Study the drawing (mm; zero at the part's minimum x, y, z) and answer. A direction names the side the tool comes from. Give positions to 0.01 mm unless a question says otherwise; leave off trailing zeros. Loops run counter-clockwise (first coordinate to the right, second up) from the corner with the lowest first, then second, coordinate; pieces in that order, holes last. Notation, with made-up numbers: (-21, -18) - (28, -18) arc R16 cw to (28, 10) - close; hole circle Ø2 at (-9.75, 46.25). An arc over 180 degrees is marked (long way). Answer in a Markdown table with one row per item. Add a question column.
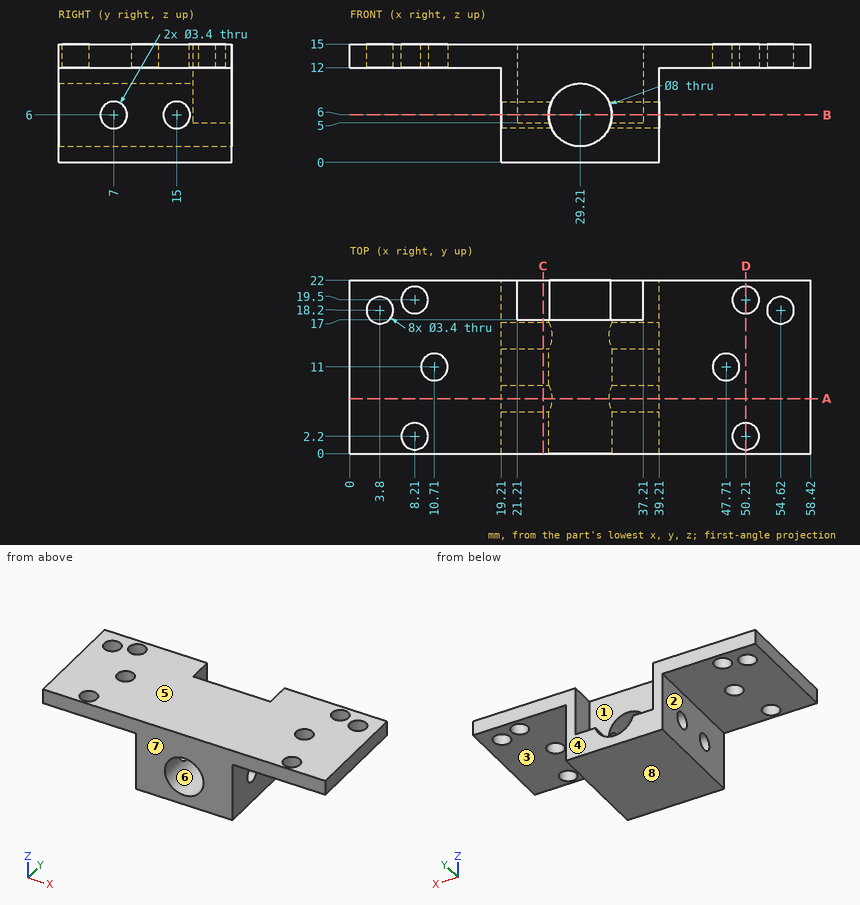
(1) A tool of negligible diameter and unlimited length cuts with its end or side. For the marked faces 1, 2, 3 and 4, from which of +Z, -Z, +X, -X, +Y, -Y can it reach the whole face along a straight path? Write none if from no direction.
(2) The mould has two halves that part along Z. Classify the marked faces 5, 6, 7 and 8: pulls with the +Z half, pulls with the -Z half, needs draft (parallel to the pull), parting line crosses it, or undercut.
(3) A cutting plane is placed at C-C on x = 24.5. Determine the outline of the cut face in (y, z), plus the area to 3 significant figures.
(4) A cutting plane is placed at B-B on z = 6. Determine the outline of the cut face in (x, y), plus the area to 3 significant figures.
(5) A cutting plane is placed at A-A on y = 7. Determine the outline of the cut face in (x, z).
(6) Find the intervals of material crossed by line 1 along Y through (x, z) = (21.5, 6); line 2 along Y through (x, z) = (8.21, 13.35); line 3 along Y through (x, z) = (3.8, 13.5), in increasing order. Write a range as [from, to].
(7) A cutting plane is placed at D-D on x = 50.21. Determine the outline of the cut face in (y, z).
(8) Given pin 1 Ø8 at (x, z) = (28.5, 9.5) entering from +Y; pin 2 Ø4 at (x, y) = (47.71, 11) entering from -Z; pin 3 Ø4 at (y, z) = (2.5, 3) entering from +X, each flat-ended and moving along its own axis, determine where each tip first touches the part or whether it passes through.
Evaluation:
| question | item | result |
|---|---|---|
| 1 | face 1 | +Z, +Y |
| 1 | face 2 | -Z, -X, +Y, -Y |
| 1 | face 3 | -Z, +X, +Y, -Y |
| 1 | face 4 | +Z, -Z, +X, -X, +Y |
| 2 | face 5 | pulls with the +Z half |
| 2 | face 6 | undercut |
| 2 | face 7 | needs draft |
| 2 | face 8 | pulls with the -Z half |
| 3 | outline | (0, 0) - (22, 0) - (22, 5) - (17, 5) - (17, 15) - (0, 15) - close; hole circle Ø3.4 at (7, 6); hole circle Ø3.4 at (15, 6) |
| 3 | area | 262 mm² |
| 4 | outline | (19.21, 0) - (25.21, 0) - (25.21, 5.3) - (19.21, 5.3) - close; (19.21, 8.7) - (25.21, 8.7) - (25.21, 13.3) - (19.21, 13.3) - close; (19.21, 16.7) - (25.21, 16.7) - (25.21, 17) - (21.21, 17) - (21.21, 22) - (19.21, 22) - close; (33.21, 0) - (39.21, 0) - (39.21, 5.3) - (33.21, 5.3) - close; (33.21, 8.7) - (39.21, 8.7) - (39.21, 13.3) - (33.21, 13.3) - close; (33.21, 16.7) - (39.21, 16.7) - (39.21, 22) - (37.21, 22) - (37.21, 17) - (33.21, 17) - close |
| 4 | area | 142 mm² |
| 5 | outline | (0, 12) - (19.21, 12) - (19.21, 7.7) - (25.59, 7.7) arc R4 cw to (32.83, 7.7) - (39.21, 7.7) - (39.21, 12) - (58.42, 12) - (58.42, 15) - (0, 15) - close; (19.21, 0) - (39.21, 0) - (39.21, 4.3) - (32.83, 4.3) arc R4 cw to (25.59, 4.3) - (19.21, 4.3) - close |
| 6 | line 1 | y = [0, 5.3], [8.7, 13.3], [16.7, 17] |
| 6 | line 2 | y = [0, 0.5], [3.9, 17.8], [21.2, 22] |
| 6 | line 3 | y = [0, 16.5], [19.9, 22] |
| 7 | outline | (0, 12) - (0.5, 12) - (0.5, 15) - (0, 15) - close; (3.9, 12) - (17.8, 12) - (17.8, 15) - (3.9, 15) - close; (21.2, 12) - (22, 12) - (22, 15) - (21.2, 15) - close |
| 8 | pin 1 | stops at y = 17 |
| 8 | pin 2 | stops at z = 12 |
| 8 | pin 3 | stops at x = 39.21 |
